Geometry: see drawing. Coordinates: mm, zero at the bounding-box minimum. Coordinates: 2 decimals unless noted, no trailing zeros. Order: outer loops, then holes, each group sorted by start corner. A loop starts at its lowest first (then second) coordinate and runs counter-clockwise, first axis right, second up. Notation, with made-up numbers: M -14.75,43 L -0.75,43 A13 cw -0.75,53 Z; hole C 74.25,52 d1. An arc over 180 degrees is marked long. One line per item, written item: value.
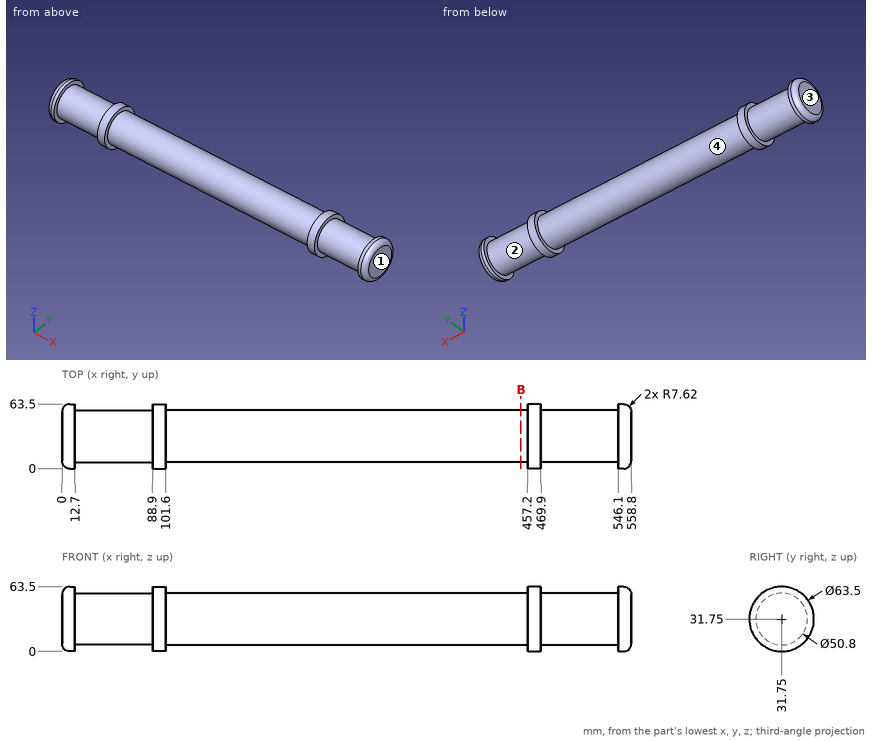
(1) Cut plane B-B on x = 450.5. Output: boundary loops of the cut face in (y, z).
Data:
outline: C 31.75,31.75 d50.8
(2) Ray query, line 1 (X direction, y = 51, z = 9); line 2 (X direction, y = 30.5, z = 59); line 3 (Z direction, x = 254, y = 32). Return the intervals inside material, ascending. Write a range as from..to.
Data:
line 1: x = 2.53..12.7, 88.9..101.6, 457.2..469.9, 546.1..556.27
line 2: x = 0.68..12.7, 88.9..101.6, 457.2..469.9, 546.1..558.12
line 3: z = 6.35..57.15
(3) Draft query along X for the marked faces 1, 2, 3 and 4. Return one class per face: released by +X, released by -X, zero draft, split by the parting line, or undercut.
Data:
face 1: released by +X
face 2: undercut
face 3: released by -X
face 4: undercut
(4) First-contact query: pin 1 (10 mm diameter, centred on x = 445, z = 46.5, fed in from -Y); pin 2 (5 mm diameter, centred on y = 52.5, z = 53, fed in from +X); pin 3 (5 mm diameter, centred on x = 395.5, y = 39, fed in from -Z). Flat tips, straight axial feed; report the tip coordinate or a pass-through.
Data:
pin 1: stops at y = 8.3
pin 2: stops at x = 558.15
pin 3: stops at z = 6.8
